```python
from build123d import *

# Parameters (mm, degrees)
PAD_DEPTH = 5
BOX_W     = 17.99
BOX_H     = 15
BOX_DEPTH = 10


with BuildPart() as obj1:
    # Sketch → Pad (new body)
    with BuildSketch(Plane(origin=(0, 0, 0), x_dir=(-1, 0, 0), z_dir=(0, 0, 1))):
        Polygon((0, 0), (0, -12), (-17.994986, -7.5), (-17.994986, 0), align=None)
    extrude(amount=PAD_DEPTH)


with BuildPart() as f_150mm:
    # Box → Box (new body)
    with BuildSketch(Plane(origin=(0, -2, 0), x_dir=(1, 0, 0), z_dir=(0, 0, 1))):
        with Locations((8.995, 7.5)):
            Rectangle(BOX_W, BOX_H)
    extrude(amount=BOX_DEPTH)

    # Cut: cut obj1
    add(obj1.part, mode=Mode.SUBTRACT)


solid = f_150mm.part
```
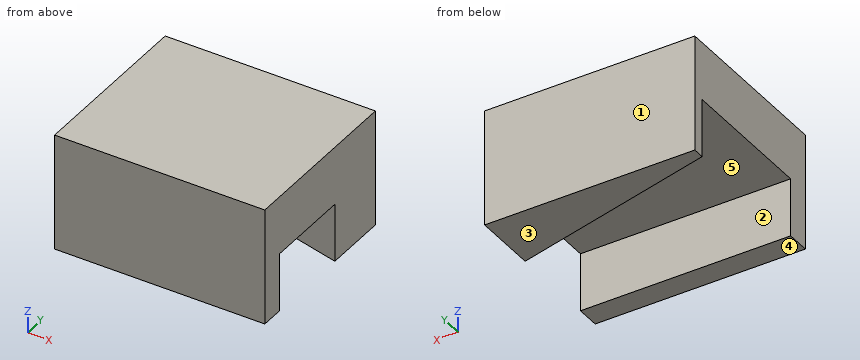
Work out the finished part from the listing and answer in its coordinate system (mm). Face numbers are marked on the shaded views. A direction names the side the tool comes from. Coordinates: 2 decimals unless noted, no trailing zeros. Order: outer loops, then holes, each group sorted by start corner. A loop starts at its lowest first (then second) coordinate and runs counter-clockwise, first axis right, second up. Notation, with made-up numbers: (51, -5) - (65, -5) arc R25 ccw to (65, 9) - close; hole circle Ø10 at (63, 37). An arc over 180 degrees is marked (long way). Answer as a JSON object with one key per item and string values.
1. The mould has two halves that part along Y. Classify the marked faces 1, 2 and 3: +Y half, -Y half, draft (parallel to the pull), parting line (faces both ways), or undercut.
Output values:
{"face 1": "+Y half", "face 2": "undercut", "face 3": "draft"}
2. Consider line 1 (Z direction, x = 13, y = 8); line 2 (Y direction, x = 12, z = 1); line 3 (Y direction, x = 4.75, z = 2.5). Determine where each line is inside the solid, lowest interval first.
Output values:
{"line 1": "z = 5 to 10", "line 2": "y = -2 to 0, 9 to 13", "line 3": "y = -2 to 0, 10.81 to 13"}
3. This flat-tipped pin is pushed along its axis until it touches: P1, Ø6, axis at x = 15, y = 0.5, coming from the -Z side. Where does it stop, or does it pass through?
Output values:
{"P1": "stops at z = 0"}
4. Find section B-B on x = 3.25. Determine the outline of the cut face in (y, z), plus the area to 3 significant figures.
Output values:
{"outline": "(-2, 0) - (0, 0) - (0, 5) - (11.19, 5) - (11.19, 0) - (13, 0) - (13, 10) - (-2, 10) - close", "area": "94.1 mm²"}
5. Find section D-D on x = 12.5. Determine the outline of the cut face in (y, z), plus the area to 3 significant figures.
Output values:
{"outline": "(-2, 0) - (0, 0) - (0, 5) - (8.87, 5) - (8.87, 0) - (13, 0) - (13, 10) - (-2, 10) - close", "area": "106 mm²"}
6. Find section A-A on z = 1.25. Determine the outline of the cut face in (x, y), plus the area to 3 significant figures.
Output values:
{"outline": "(0, -2) - (17.99, -2) - (17.99, 0) - (0, 0) - close; (0, 12) - (17.99, 7.5) - (17.99, 13) - (0, 13) - close", "area": "94.4 mm²"}
7. Find section C-C on y = 2. Determine the outline of the cut face in (x, z), plus the area to 4 significant figures.
Output values:
{"outline": "(0, 5) - (17.99, 5) - (17.99, 10) - (0, 10) - close", "area": "89.95 mm²"}
8. A tool of negligible diameter and unlimited length cuts with its end or side. For the marked faces 4 and 5, from which of +Z, -Z, +X, -X, +Y, -Y can it reach the whole face along a straight path? Write none if from no direction.
Output values:
{"face 4": "-Z, +X, -X, +Y, -Y", "face 5": "-Z, -X"}
